Check sheet for the modelled part. Datum: model origin and axes. Units: mm. Give positions to 0.01 mm unless a question says otherwise; leave off trailing zeros.
Item 1: Gauge pin test, flat ends, axial feed: P1, Ø0.9, axis at x = 1, y = 16, coming from the -Z side; P2, Ø0.9, axis at x = 1.5, z = 3.5, coming from the +Y side; P3, Ø0.9, axis at x = 2, z = 3.5, coming from the -Y side. Record the tip position at first contact, or that the pin passes through.
Item 2: Sectioned sample at A-A on z = 1.5. Count the separate pieces of the cut face and the enclosed holes in it, and give its area (3 significant figures).
Item 3: Material ranges on line 1 along Z through (x, y) = (0.3, 112), recorded low to high.
from build123d import *

# Parameters (mm, degrees)
F0_W     = 1.5
F0_H     = 5
F0_W_2   = 3
F1_DEPTH = 3


with BuildPart() as f1:
    # F0 (on Right) → F1 (new body)
    with BuildSketch(Plane.YZ):
        Polygon((1.5, 5), (1.5, 0), (11.5, 0), (14.5, 0), (14.5, 5), (14.5, 10), (11.5, 10), (1.5, 10), align=None)
        Polygon((17.5, 5), (17.5, 0), (20.5, 0), (30.5, 0), (30.5, 5), (30.5, 10), (20.5, 10), (17.5, 10), align=None)
        with Locations((0.75, 7.5)):
            Rectangle(F0_W, F0_H)
        with Locations((-0.75, 7.5)):
            Rectangle(F0_W, F0_H)
        with Locations((16, 7.5)):
            Rectangle(F0_W_2, F0_H)
        with Locations((32, 7.5)):
            Rectangle(F0_W_2, F0_H)
        with Locations((48, 7.5)):
            Rectangle(F0_W_2, F0_H)
        with Locations((64, 7.5)):
            Rectangle(F0_W_2, F0_H)
        with Locations((80, 7.5)):
            Rectangle(F0_W_2, F0_H)
        with Locations((95.25, 7.5)):
            Rectangle(F0_W, F0_H)
        with Locations((96.75, 7.5)):
            Rectangle(F0_W, F0_H)
        with Locations((112, 7.5)):
            Rectangle(F0_W_2, F0_H)
        with Locations((128, 7.5)):
            Rectangle(F0_W_2, F0_H)
        with Locations((144, 7.5)):
            Rectangle(F0_W_2, F0_H)
        with Locations((160, 7.5)):
            Rectangle(F0_W_2, F0_H)
        with Locations((176, 7.5)):
            Rectangle(F0_W_2, F0_H)
        with Locations((191.25, 7.5)):
            Rectangle(F0_W, F0_H)
        with Locations((192.75, 7.5)):
            Rectangle(F0_W, F0_H)
        Polygon((33.5, 5), (33.5, 0), (43.5, 0), (46.5, 0), (46.5, 5), (46.5, 10), (33.5, 10), align=None)
        Polygon((49.5, 5), (49.5, 0), (52.5, 0), (62.5, 0), (62.5, 5), (62.5, 10), (49.5, 10), align=None)
        Polygon((78.5, 10), (65.5, 10), (65.5, 5), (65.5, 0), (75.5, 0), (78.5, 0), (78.5, 5), align=None)
        Polygon((94.5, 10), (81.5, 10), (81.5, 5), (81.5, 0), (84.5, 0), (94.5, 0), (94.5, 5), align=None)
        Polygon((110.5, 10), (97.5, 10), (97.5, 5), (97.5, 0), (107.5, 0), (110.5, 0), (110.5, 5), align=None)
        Polygon((126.5, 10), (113.5, 10), (113.5, 5), (113.5, 0), (116.5, 0), (126.5, 0), (126.5, 5), align=None)
        Polygon((142.5, 10), (129.5, 10), (129.5, 5), (129.5, 0), (139.5, 0), (142.5, 0), (142.5, 5), align=None)
        Polygon((158.5, 10), (145.5, 10), (145.5, 5), (145.5, 0), (148.5, 0), (158.5, 0), (158.5, 5), align=None)
        Polygon((171.5, 10), (161.5, 10), (161.5, 5), (161.5, 0), (171.5, 0), (174.5, 0), (174.5, 5), (174.5, 10), align=None)
        Polygon((180.5, 10), (177.5, 10), (177.5, 5), (177.5, 0), (180.5, 0), (190.5, 0), (190.5, 5), (190.5, 10), align=None)
    extrude(amount=F1_DEPTH)


solid = f1.part
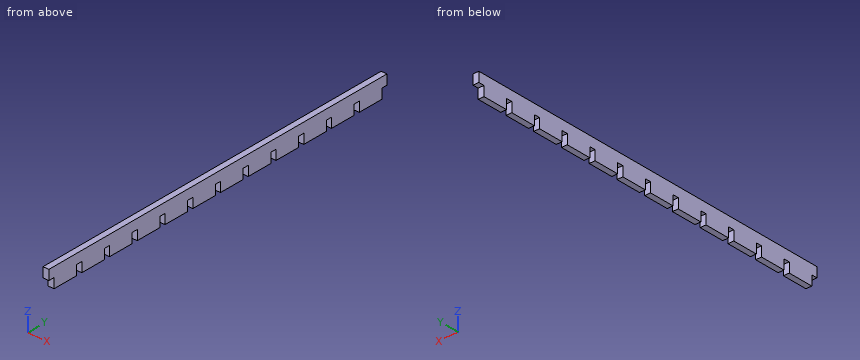
Report:
1. P1: stops at z = 5
1. P2: stops at y = 190.5
1. P3: stops at y = 1.5
2. separate pieces: 12
2. enclosed holes: 0
2. area: 468 mm2
3. line 1: z = 5 to 10
